from build123d import *

# Parameters (mm, degrees)
SKETCH1_W           = 552.45
SKETCH1_H           = 19.05
SKETCH1_R           = 5.588
BOSS_EXTRUDE1_DEPTH = 6.35
FILLET1_R           = 2.54


with BuildPart() as part:
    # Sketch1 → Boss-Extrude1 (new, symmetric)
    with BuildSketch(Plane.XY):
        Rectangle(SKETCH1_W, SKETCH1_H)
        Circle(SKETCH1_R, mode=Mode.SUBTRACT)
        with Locations((-250.825, 0)):
            Circle(SKETCH1_R, mode=Mode.SUBTRACT)
        with Locations((250.825, 0)):
            Circle(SKETCH1_R, mode=Mode.SUBTRACT)
    extrude(amount=BOSS_EXTRUDE1_DEPTH, both=True)

    # Fillet1
    fillet1_edges = [part.edges().sort_by_distance(p)[0] for p in [
        (276.225, -9.525, 0),
        (-276.225, -9.525, 0),
        (-276.225, 9.525, 0),
        (276.225, 9.525, 0),
    ]]
    fillet(fillet1_edges, radius=FILLET1_R)


solid = part.part
Could you check a few things on this model? Use its own coordinates, in mm. Round coordinates to 2 decimals unless told otherwise and drop trailing zeros. Loops run counter-clockwise (first coordinate to the right, second up) from the corner with the lowest first, then second, coordinate; pieces in that order, holes last. Notation, with made-up numbers: (38.5, 71.5) -> (81.5, 71.5) arc R30 cw to (81.5, 94.5) -> close; hole circle Ø2 at (38, 61.5). An arc over 180 degrees is marked (long way). Use CSV: the item, a comma, the result in double quotes.
(1) Will this pin go through, and if not, where does the flat tip stop? pin 1 Ø10 at (x, y) = (250.825, 0) entering from +Z.
Return value:
pin 1,"passes through"
(2) Suppose I cut it at A-A on z = 1.25. Write out the boundary of the cut face in (x, y) (3 decimals), plus the area to 3 significant figures.
Return value:
outline,"(-276.225, -6.985) arc R2.54 ccw to (-273.685, -9.525) -> (273.685, -9.525) arc R2.54 ccw to (276.225, -6.985) -> (276.225, 6.985) arc R2.54 ccw to (273.685, 9.525) -> (-273.685, 9.525) arc R2.54 ccw to (-276.225, 6.985) -> close; hole circle Ø11.176 at (-250.825, 0); hole circle Ø11.176 at (0, 0); hole circle Ø11.176 at (250.825, 0)"
area,"10,200 mm²"
(3) If we mould it in two halves opening along Y, with no side actions, what happens to faces 1 (the flat face through (-4, 9.525, 0)), 2 (the flat face through (-276.225, 0, 0)), 3 (the cylindrical face through (246.71, 3.78, -0.09))? For each: +Y half, -Y half, draft (parallel to the pull), parting line (faces both ways), or undercut.
Return value:
face 1,"+Y half"
face 2,"draft"
face 3,"undercut"
(4) Suppose I cut it at B-B on x = 0. Write out the boundary of the cut face in (y, z) (3 decimals).
Return value:
outline,"(-9.525, -6.35) -> (-5.588, -6.35) -> (-5.588, 6.35) -> (-9.525, 6.35) -> close; (5.588, -6.35) -> (9.525, -6.35) -> (9.525, 6.35) -> (5.588, 6.35) -> close"
(5) If I drill on probe 1 along X at (y, z) = (-0.5, -5.25) (3 decimals); probe 2 along X at (y, z) = (0.75, 3.25) (3 decimals); probe 3 along Y at (x, z) = (-253.5, -3.75) (3 decimals), over which ranges is the centre line in solid material (lowest first)? Write a range as [from, to].
Return value:
probe 1,"x = [-276.225, -256.391], [-245.259, -5.566], [5.566, 245.259], [256.391, 276.225]"
probe 2,"x = [-276.225, -256.362], [-245.288, -5.537], [5.537, 245.288], [256.362, 276.225]"
probe 3,"y = [-9.525, -4.906], [4.906, 9.525]"
